Part model, mm, in its own coordinate system. Round coordinates to 2 decimals unless told otherwise and drop trailing zeros. Order: outer loops, then holes, each group sorted by start corner. A loop starts at its lowest first (then second) coordinate and runs counter-clockwise, first axis right, second up. Notation, with made-up numbers: M 78,79.5 L 92,79.5 A9 ccw 92,96.5 Z; hole C 80,-35.75 d10. An arc over 180 degrees is marked long. Write each question's results on one line, items separated by ' | '. Start each with the question number.
1. Probe L1, parallel to Y at x = 50.8, z = 2.5; L2, parallel to X at y = -36, z = 1.35; L3, parallel to X at y = 75, z = 2.55. List the from-to ranges inside material, lowest first. Write a range as [from, to].
2. Band-saw the part on A-A, the plane y = 38.1. List the corners of the cut face in (x, z) (3 decimals).
3. Two-plate mould, pull along X, no slides. Class faces 1 (the face through (-1, 1, 3.175)), 2 (the face through (53.377, 76.313, 1.61)): +X half, -X half, draft (parallel to the pull), parting line (faces both ways), or undercut.
4. Band-saw the part on B-B, the plane x = -50.8. List the corners of the cut face in (y, z) (3 decimals).
```python
from build123d import *

# Parameters (mm, degrees)
SKETCH1_W           = 127
SKETCH1_H           = 203.2
BOSS_EXTRUDE1_DEPTH = 3.175
SKETCH2_R           = 2.5796875
CUT_EXTRUDE1_DEPTH  = 6.35


with BuildPart() as part:
    # Sketch1 → Boss-Extrude1 (new body)
    with BuildSketch(Plane.XY):
        Rectangle(SKETCH1_W, SKETCH1_H)
    extrude(amount=BOSS_EXTRUDE1_DEPTH)

    # Sketch2 → Cut-Extrude1 (cut)
    with BuildSketch(Plane.XY.offset(3.175)):
        with Locations((-50.8, 76.2)):
            Circle(SKETCH2_R)
        with Locations((-50.8, 38.1)):
            Circle(SKETCH2_R)
        with Locations((-50.8, -38.1)):
            Circle(SKETCH2_R)
        with Locations((-50.8, -76.2)):
            Circle(SKETCH2_R)
    cut_extrude1 = extrude(amount=-CUT_EXTRUDE1_DEPTH, mode=Mode.SUBTRACT)

    # Mirror1: Cut-Extrude1 across plane
    add(cut_extrude1.mirror(Plane(origin=(0, 0, 0), x_dir=(0, 0, 1), z_dir=(1, 0, 0))), mode=Mode.SUBTRACT)


solid = part.part
```
Solution:
1) L1: [-101.6, -78.78], [-73.62, -40.68], [-35.52, 35.52], [40.68, 73.62], [78.78, 101.6] | L2: [-63.5, -52.3], [-49.3, 49.3], [52.3, 63.5] | L3: [-63.5, -53.08], [-48.52, 48.52], [53.08, 63.5]
2) outline: M -63.5,0 L -53.38,0 L -53.38,3.175 L -63.5,3.175 Z; M -48.22,0 L 48.22,0 L 48.22,3.175 L -48.22,3.175 Z; M 53.38,0 L 63.5,0 L 63.5,3.175 L 53.38,3.175 Z
3) face 1: draft | face 2: undercut
4) outline: M -101.6,0 L -78.78,0 L -78.78,3.175 L -101.6,3.175 Z; M -73.62,0 L -40.68,0 L -40.68,3.175 L -73.62,3.175 Z; M -35.52,0 L 35.52,0 L 35.52,3.175 L -35.52,3.175 Z; M 40.68,0 L 73.62,0 L 73.62,3.175 L 40.68,3.175 Z; M 78.78,0 L 101.6,0 L 101.6,3.175 L 78.78,3.175 Z
